from build123d import *

# Parameters (mm, degrees)
F0_R           = 6
F1_DEPTH       = 22
F2_DEPTH       = 10
F3_R           = 3
F5_D           = 5
F5_DEPTH       = 16
F5_CBORE_D     = 10
F5_CBORE_DEPTH = 3
F5_TIP         = 1.5021515476
F7_DEPTH       = 2
F8_D           = 6
F8_DEPTH       = 16
F8_TIP         = 1.8025818571


with BuildPart() as f1:
    # F0 (on Front) → F1 (new body)
    with BuildSketch(Plane.XZ):
        with BuildLine():
            ThreePointArc((12.7781681608, 11.6290403704), (7.1391649946, 16.3189497932), (-3.39e-08, 18))
            ThreePointArc((-3.39e-08, 18), (-7.1391650249, 16.3189497781), (-12.7781681608, 11.6290403704))
            Line((-12.7781681608, 11.6290403704), (-27.5697110315, -8))
            Line((-27.5697110315, -8), (-32, -8))
            Line((-32, -8), (-32, -18))
            Line((-32, -18), (-8, -18))
            Line((-8, -18), (-8, -27))
            Line((-8, -27), (8, -27))
            Line((8, -27), (8, -18))
            Line((8, -18), (32, -18))
            Line((32, -18), (32, -8))
            Line((32, -8), (27.5697110315, -8))
            Line((27.5697110315, -8), (12.7781681608, 11.6290403704))
        make_face()
        with Locations((0, 2)):
            Circle(F0_R, mode=Mode.SUBTRACT)
    extrude(amount=F1_DEPTH)

    # F0 (on Front) → F2 (join)
    with BuildSketch(Plane.XZ):
        with BuildLine():
            Line((32, -8), (32, 18))
            Line((32, 18), (-3.39e-08, 18))
            ThreePointArc((-3.39e-08, 18), (7.1391649946, 16.3189497932), (12.7781681608, 11.6290403704))
            Line((12.7781681608, 11.6290403704), (27.5697110315, -8))
            Line((27.5697110315, -8), (32, -8))
        make_face()
        with BuildLine():
            ThreePointArc((-12.7781681608, 11.6290403704), (-7.1391650249, 16.3189497781), (-3.39e-08, 18))
            Line((-3.39e-08, 18), (-32, 18))
            Line((-32, 18), (-32, -8))
            Line((-32, -8), (-27.5697110315, -8))
            Line((-27.5697110315, -8), (-12.7781681608, 11.6290403704))
        make_face()
        with BuildLine():
            ThreePointArc((12.7781681608, 11.6290403704), (7.1391649946, 16.3189497932), (-3.39e-08, 18))
            ThreePointArc((-3.39e-08, 18), (-7.1391650249, 16.3189497781), (-12.7781681608, 11.6290403704))
            Line((-12.7781681608, 11.6290403704), (-27.5697110315, -8))
            Line((-27.5697110315, -8), (-32, -8))
            Line((-32, -8), (-32, -18))
            Line((-32, -18), (-8, -18))
            Line((-8, -18), (-8, -27))
            Line((-8, -27), (8, -27))
            Line((8, -27), (8, -18))
            Line((8, -18), (32, -18))
            Line((32, -18), (32, -8))
            Line((32, -8), (27.5697110315, -8))
            Line((27.5697110315, -8), (12.7781681608, 11.6290403704))
        make_face()
        with Locations((0, 2)):
            Circle(F0_R, mode=Mode.SUBTRACT)
        with Locations((0, 2)):
            Circle(F0_R)
    extrude(amount=-F2_DEPTH)

    # F3
    f3_edges = [f1.edges().sort_by_distance(p)[0] for p in [
        (-27.569711, -11, -8),
        (27.569711, -11, -8),
    ]]
    fillet(f3_edges, radius=F3_R)

    # F5
    with Locations(Plane.XY.offset(18)):
        with Locations((0, -10)):
            CounterBoreHole(F5_D / 2, F5_CBORE_D / 2, F5_CBORE_DEPTH, depth=F5_DEPTH)
            with Locations((0, 0, -(F5_DEPTH + F5_TIP / 2))):  # 118° drill point
                Cone(0, F5_D / 2, F5_TIP, mode=Mode.SUBTRACT)

    # F0 (on Front) → F7 (cut)
    with BuildSketch(Plane.XZ):
        with Locations((0, 2)):
            Circle(F0_R)
    extrude(amount=-F7_DEPTH, mode=Mode.SUBTRACT)

    # F8
    with Locations(Plane(origin=(0, 0, -27), x_dir=(1, 0, 0), z_dir=(0, 0, -1))):
        with Locations((0, -2), (0, 14)):
            Hole(F8_D / 2, depth=F8_DEPTH)
            with Locations((0, 0, -(F8_DEPTH + F8_TIP / 2))):  # 118° drill point
                Cone(0, F8_D / 2, F8_TIP, mode=Mode.SUBTRACT)


solid = f1.part
Build history of the part. All positions in model axes, mm. A direction names the side the tool comes from. Coordinates: 2 decimals unless noted, no trailing zeros. Order: outer loops, then holes, each group sorted by start corner. A loop starts at its lowest first (then second) coordinate and runs counter-clockwise, first axis right, second up. Notation, with made-up numbers: (32.5, 75) - (48.5, 75) arc R20 ccw to (48.5, 102) - close; hole circle Ø10 at (-38, -28.5). An arc over 180 degrees is marked (long way). Write each question's results on one line, items separated by ' | '. Start each with the question number.
Item 1: Band-saw the part on B-B on y = -8.5. Write the cut outline in (x, z), and give its area (3 significant figures).
Item 2: Wall check: probe 1 along Y at (x, z) = (0, -21); probe 2 along Z at (x, y) = (0, -5.25); probe 3 along Y at (x, z) = (0, 11). Give the ranges that are in metal, low to high. Write a range as [from, to].
Item 3: Band-saw the part on A-A on z = -14. Write the cut outline in (x, y).
Item 4: Mould opens along Y. For faces 5 (the face through (20, -6, -18)), 6 (the face through (0, 2, 2)), 7 (the face through (2.5, -9.9, 11.2)), 8 (the face through (0.65, -11.07, -18.89)) say: released by +Y, released by -Y, zero draft, split by the parting line, or undercut.
Item 5: Band-saw the part on C-C on x = -13.5. Write the cut outline in (y, z).
Item 6: Flat gauge pins, fed straight in: pin 1 (2 mm diameter, centred on y = -2.5, z = 3, fed in from +X); pin 2 (10 mm diameter, centred on y = -10, z = -24.5, fed in from -X); pin 3 (6 mm diameter, centred on x = 0, y = -10, fed in from +Z). Where does each tip first touch, or does it go through?
Item 7: Band-saw the part on D-D on z = -20.5. Write the cut outline in (x, y).
Item 8: Tool access for faces 1 (the face through (0.65, 4.93, -18.89)), 2 (the face through (-20, -6, -18)), 3 (the face through (-1.301, -9.832, -3.857)), 4 (the face through (-23, 0, 8)): list every direction of +Z, -Z, +X, -X, +Y, -Y with a clear straight run to the whole face (end or side of a thin tool).
Numbers:
1) outline: (-32, -18) - (-8, -18) - (-8, -27) - (8, -27) - (8, -18) - (32, -18) - (32, -8) - (29.07, -8) arc R3 cw to (26.67, -6.81) - (12.78, 11.63) arc R16 ccw to (4.77, 17.27) - (4.77, 15) - (2, 15) - (2, 7.66) arc R6 cw (long way) to (-2, 7.66) - (-2, 15) - (-4.77, 15) - (-4.77, 17.27) arc R16 ccw to (-12.78, 11.63) - (-26.67, -6.81) arc R3 cw to (-29.07, -8) - (-32, -8) - close | area: 1,520 mm^2
2) probe 1: [-22, -17], [-11, -1], [5, 10] | probe 2: [-27, -4], [8, 15] | probe 3: [-22, -12.5], [-7.5, 10]
3) outline: (-32, -22) - (32, -22) - (32, 10) - (-32, 10) - close; hole circle Ø6 at (0, -14); hole circle Ø6 at (0, 2)
4) face 5: zero draft | face 6: released by -Y | face 7: undercut | face 8: undercut
5) outline: (-22, -18) - (10, -18) - (10, 18) - (0, 18) - (0, 10.67) - (-22, 10.67) - close
6) pin 1: x = 20.03 | pin 2: x = -8 | pin 3: z = 15
7) outline: (-8, -22) - (8, -22) - (8, 10) - (-8, 10) - close; hole circle Ø6 at (0, -14); hole circle Ø6 at (0, 2)
8) face 1: -Z | face 2: -Z, -X, +Y, -Y | face 3: -Y | face 4: +Z, -X, -Y
